```python
from build123d import *

# Parameters (mm, degrees)
F0_R     = 27.5
F1_DEPTH = 38.1
F2_W     = 19.05
F2_H     = 5.08
F3_DEPTH = 38.1
F5_D     = 6.7564


with BuildPart() as f1:
    # F0 (on Front) → F1 (new body)
    with BuildSketch(Plane.XZ):
        Polygon((-44.45, 0), (0, 0), (44.45, 0), (44.45, 17.78), (41.275, 19.05), (41.275, 52.07), (26.035, 52.07), (13.97, 66.04), (0, 66.04), (-13.97, 66.04), (-26.035, 52.07), (-41.275, 52.07), (-41.275, 19.05), (-44.45, 17.78), align=None)
        with Locations((0, 32.19)):
            Circle(F0_R, mode=Mode.SUBTRACT)
    extrude(amount=F1_DEPTH)

    # F2 (on face) → F3 (cut, through all)
    with BuildSketch(Plane.XZ.offset(38.1)):
        with Locations((-31.75, 34.29)):
            Rectangle(F2_W, F2_H)
    extrude(amount=-F3_DEPTH, mode=Mode.SUBTRACT)

    # F5 (through all)
    with Locations(Plane.XY.offset(52.07)):
        with Locations((-34.925, -8.89), (-34.925, -29.21), (34.925, -8.89), (34.925, -29.21)):
            Hole(F5_D / 2)


solid = f1.part
```
Design review of the part built by this model. Coordinates are the model's own, in mm. A direction names the side the tool comes from. Coordinates: 2 decimals unless noted, no trailing zeros. Write each loop counter-clockwise with the first axis right and the second up, starting at its lowest first coordinate (ties: lowest second). Pieces come first, ordered by that corner, then holes.
1) Machinability: for faces 1 (the flat face through (41.275, -19, 35)), 2 (the flat face through (-34, -19, 52.07)), 3 (the flat face through (-34, -19, 31.75)), which of the approach directions +Z, -Z, +X, -X, +Y, -Y give a long, thin tool a straight path to every point of the face, cutting with its end or side? Answer none if there is none.
2) Add section B-B (y = -8.89). Write out the cut boundary in (x, z) (3 decimals).
3) Mouldability with a two-part tool opening along X and no side actions: class faces 4 (the flat face through (34, -19, 52.07)), 5 (the cylindrical face through (-34.193, -32.508, 44.343)), 6 (the flat face through (-41.275, -19, 25)) as +X half, -X half, draft (parallel to the pull), parting line (faces both ways), or undercut.
4) Add section D-D (x = -35.5). Write out the cut boundary in (y, z).
5) Insertion check: pin 1 (15.5 mm diameter, centred on x = -37, y = -24.5, fed in from -Z); pin 2 (10 mm diameter, centred on y = -17.5, z = 28, fed in from -X) (3 decimals); pin 3 (9 mm diameter, centred on x = -34.925, y = -29.21, fed in from +Z); pin 4 (8 mm diameter, centred on y = -17.5, z = 54.5, fed in from +X) (3 decimals). Each pin has a flat end and moves straight along its axis. Give the tip position at first contact, or say it passes through.
6) Add section C-C (z = 29). Write out the cut boundary in (x, y) (3 decimals), plus the area to 3 significant figures.
7) To check wall thickness, follow L1, parallel to X at y = -29, z = 41 (3 decimals); L2, parallel to X at y = -8, z = 46 (3 decimals); L3, parallel to Y at x = 37, z = 45. State the ranges of each line that lie inside material, in increasing order.
8) Add section A-A (x = 0). Write out the cut boundary in (y, z).
Check result:
1. face 1: +Z, +X, +Y, -Y
1. face 2: +Z, -X, +Y, -Y
1. face 3: -X, +Y, -Y
2. outline: (-44.45, 0) - (-38.303, 0) - (-38.303, 31.75) - (-41.275, 31.75) - (-41.275, 19.05) - (-44.45, 17.78) - close; (-41.275, 36.83) - (-38.303, 36.83) - (-38.303, 52.07) - (-41.275, 52.07) - close; (-31.547, 0) - (31.547, 0) - (31.547, 52.07) - (26.035, 52.07) - (13.97, 66.04) - (-13.97, 66.04) - (-26.035, 52.07) - (-31.547, 52.07) - (-31.547, 36.83) - (-27.106, 36.83) arc R27.5 cw (long way) to (-27.496, 31.75) - (-31.547, 31.75) - close; (38.303, 0) - (44.45, 0) - (44.45, 17.78) - (41.275, 19.05) - (41.275, 52.07) - (38.303, 52.07) - close
3. face 4: draft
3. face 5: undercut
3. face 6: -X half
4. outline: (-38.1, 0) - (-32.54, 0) - (-32.54, 31.75) - (-38.1, 31.75) - close; (-38.1, 36.83) - (-32.54, 36.83) - (-32.54, 52.07) - (-38.1, 52.07) - close; (-25.88, 0) - (-12.22, 0) - (-12.22, 31.75) - (-25.88, 31.75) - close; (-25.88, 36.83) - (-12.22, 36.83) - (-12.22, 52.07) - (-25.88, 52.07) - close; (-5.56, 0) - (0, 0) - (0, 31.75) - (-5.56, 31.75) - close; (-5.56, 36.83) - (0, 36.83) - (0, 52.07) - (-5.56, 52.07) - close
5. pin 1: stops at z = 0
5. pin 2: stops at x = -41.275
5. pin 3: stops at z = 52.07
5. pin 4: stops at x = 41.275
6. outline: (-41.275, -38.1) - (-27.314, -38.1) - (-27.314, 0) - (-41.275, 0) - close; (27.314, -38.1) - (41.275, -38.1) - (41.275, 0) - (27.314, 0) - close; hole circle Ø6.756 at (-34.925, -29.21); hole circle Ø6.756 at (-34.925, -8.89); hole circle Ø6.756 at (34.925, -29.21); hole circle Ø6.756 at (34.925, -8.89)
6. area: 920 mm2
7. L1: x = -41.275 to -38.297, -31.553 to -26.051, 26.051 to 31.553, 38.297 to 41.275
7. L2: x = -41.275 to -38.184, -31.666 to -23.781, 23.781 to 31.666, 38.184 to 41.275
7. L3: y = -38.1 to -31.88, -26.54 to -11.56, -6.22 to 0
8. outline: (-38.1, 0) - (0, 0) - (0, 4.69) - (-38.1, 4.69) - close; (-38.1, 59.69) - (0, 59.69) - (0, 66.04) - (-38.1, 66.04) - close
